The listing builds one solid part. Answer for the finished solid, in the listing's coordinates (mm). A direction names the side the tool comes from. Coordinates: 2 decimals unless noted, no trailing zeros. Loops run counter-clockwise (first coordinate to the right, second up) from the corner with the lowest first, then second, coordinate; pieces in that order, holes last. Notation, with made-up numbers: M 23,2 L 43,2 A22 cw 43,27 Z; hole C 88.5,27 d10. An arc over 180 degrees is marked long. Return JSON: item names as keys, results as strings. Group by question number.
1. Section A-A (z = 1.75) is taken. Write down the section's boundary in (x, y), then the cut area to 3 significant figures.
2. Which of the six approach directions +Z, -Z, +X, -X, +Y, -Y give full straight-line access (tool end or side, diameter ignored) to faces 1 (the face through (-83.949, 183.214, 5.239)), 2 (the face through (-84, 172.928, 6)), 3 (the face through (-82, 197.928, 6))?
3. Given P1, Ø5, axis at x = 86, z = 5.5, coming from the +Y side; P2, Ø2.5, axis at x = 46.78, y = 179.93, coming from the -Z side; P3, Ø5.5, axis at x = -53.42, y = 179.93, coming from the +Z side; P4, Ø0.9, axis at y = 171.5, z = 3.5, coming from the -X side, each flat-ended and moving along its own axis, determine where each tip first touches the part or whether it passes through.
4. Straight lines are drawn through the part: L1, parallel to Y at x = -83, z = 6; L2, parallel to Y at x = 19.5, z = 10.25; L3, parallel to X at y = 179, z = 6. For each, find the intervals that lie inside material, in ascending order. Write a range as from..to.
5. The mould has two halves that part along Y. Classify faces 4 (the face through (-78.019, 171, 6)), 5 (the face through (85, 197.928, 6)), 6 (the face through (87.311, 186.122, 5.785)): pulls with the +Y half, pulls with the -Y half, needs draft (parallel to the pull), parting line crosses it, or undercut.
```python
from build123d import *

# Parameters (mm, degrees)
ESBO_O1_W                                      = 119
ESBO_O1_H                                      = 30
RESSALTO_EXTRUS_O1_DEPTH                       = 12
ESCAREADO_PARA_SFHCS_M31_D                     = 3.4
ESCAREADO_PARA_SFHCS_M31_CSINK_D               = 6.72
ESCAREADO_PARA_SFHCS_M31_CSINK_ANGLE           = 90
ESBO_O8_W                                      = 26.2
ESBO_O8_H                                      = 30
RESSALTO_EXTRUS_O2_DEPTH                       = 12
ESBO_O9_W                                      = 36.2
ESBO_O9_H                                      = 30
RESSALTO_EXTRUS_O3_DEPTH                       = 12
ESBO_O10_W                                     = 12
ESBO_O10_H                                     = 12
CORTE_EXTRUS_O1_DEPTH                          = 2
FILETE1_R                                      = 2
ESBO_O12_W                                     = 11
ESBO_O12_H                                     = 12
CORTE_EXTRUS_O2_DEPTH                          = 3
BROCA_DE_ROSQUEAR_PARA_TARRAXA_DE_M4X0_7_D     = 3.3
BROCA_DE_ROSQUEAR_PARA_TARRAXA_DE_M4X0_7_DEPTH = 10
BROCA_DE_ROSQUEAR_PARA_TARRAXA_DE_M4X0_7_TIP   = 0.991420021
ESBO_O15_W                                     = 12
ESBO_O15_H                                     = 12
CORTE_EXTRUS_O3_DEPTH                          = 2
FILETE2_R                                      = 2
BROCA_DE_ROSQUEAR_PARA_TARRAXA_DE_M4_2_D       = 3.3
BROCA_DE_ROSQUEAR_PARA_TARRAXA_DE_M4_2_DEPTH   = 10
BROCA_DE_ROSQUEAR_PARA_TARRAXA_DE_M4_2_TIP     = 0.991420021


with BuildPart() as part:
    # Esboço1 → Ressalto-extrusão1 (new body)
    with BuildSketch(Plane.XY):
        with Locations((-3.319388577, 184.927849727)):
            Rectangle(ESBO_O1_W, ESBO_O1_H)
    extrude(amount=RESSALTO_EXTRUS_O1_DEPTH)

    # Escareado para SFHCS M31 (through all)
    with Locations(Plane.XY.offset(12)):
        with Locations((46.780611423, 179.927849727), (-53.419388577, 179.927849727), (-26.219388577, 179.927849727), (19.580611423, 179.927849727)):
            CounterSinkHole(ESCAREADO_PARA_SFHCS_M31_D / 2, ESCAREADO_PARA_SFHCS_M31_CSINK_D / 2, counter_sink_angle=ESCAREADO_PARA_SFHCS_M31_CSINK_ANGLE)

    # Esboço8 → Ressalto-extrusão2 (add)
    with BuildSketch(Plane.XY.offset(12)):
        with Locations((-75.919388577, 184.927849727)):
            Rectangle(ESBO_O8_W, ESBO_O8_H)
    extrude(amount=-RESSALTO_EXTRUS_O2_DEPTH)

    # Esboço9 → Ressalto-extrusão3 (add)
    with BuildSketch(Plane.XY):
        with Locations((74.280611423, 184.927849727)):
            Rectangle(ESBO_O9_W, ESBO_O9_H)
    extrude(amount=RESSALTO_EXTRUS_O3_DEPTH)

    # Esboço10 → Corte-extrusão1 (cut)
    with BuildSketch(Plane(origin=(0, 199.927849727, 0), x_dir=(1, 0, 0), z_dir=(0, 1, 0))):
        with Locations((-83.019388577, -6)):
            Rectangle(ESBO_O10_W, ESBO_O10_H)
    extrude(amount=-CORTE_EXTRUS_O1_DEPTH, mode=Mode.SUBTRACT)

    # Filete1
    filete1_edges = [part.edges().sort_by_distance(p)[0] for p in [
        (-89.019388577, 197.927849727, 6),
    ]]
    fillet(filete1_edges, radius=FILETE1_R)

    # Esboço12 → Corte-extrusão2 (cut)
    with BuildSketch(Plane.XZ.offset(-169.927849727)):
        with Locations((-83.519388577, 6)):
            Rectangle(ESBO_O12_W, ESBO_O12_H)
    extrude(amount=-CORTE_EXTRUS_O2_DEPTH, mode=Mode.SUBTRACT)

    # Broca de rosquear para tarraxa de M4x0.7
    with Locations(Plane.ZY.offset(89.019388577)):
        with Locations((6, 184.677849727)):
            Hole(BROCA_DE_ROSQUEAR_PARA_TARRAXA_DE_M4X0_7_D / 2, depth=BROCA_DE_ROSQUEAR_PARA_TARRAXA_DE_M4X0_7_DEPTH)
            with Locations((0, 0, -(BROCA_DE_ROSQUEAR_PARA_TARRAXA_DE_M4X0_7_DEPTH + BROCA_DE_ROSQUEAR_PARA_TARRAXA_DE_M4X0_7_TIP / 2))):  # 118° drill point
                Cone(0, BROCA_DE_ROSQUEAR_PARA_TARRAXA_DE_M4X0_7_D / 2, BROCA_DE_ROSQUEAR_PARA_TARRAXA_DE_M4X0_7_TIP, mode=Mode.SUBTRACT)

    # Esboço15 → Corte-extrusão3 (cut)
    with BuildSketch(Plane(origin=(0, 199.927849727, 0), x_dir=(-1, 0, 0), z_dir=(0, 1, 0))):
        with Locations((-86.380611423, 6)):
            Rectangle(ESBO_O15_W, ESBO_O15_H)
    extrude(amount=-CORTE_EXTRUS_O3_DEPTH, mode=Mode.SUBTRACT)

    # Filete2
    filete2_edges = [part.edges().sort_by_distance(p)[0] for p in [
        (92.380611423, 197.927849727, 6),
    ]]
    fillet(filete2_edges, radius=FILETE2_R)

    # Broca de rosquear para tarraxa de M4 2
    with Locations(Plane(origin=(92.380611423, 0, 0), x_dir=(0, 0, -1), z_dir=(1, 0, 0))):
        with Locations((-6, 184.4862903)):
            Hole(BROCA_DE_ROSQUEAR_PARA_TARRAXA_DE_M4_2_D / 2, depth=BROCA_DE_ROSQUEAR_PARA_TARRAXA_DE_M4_2_DEPTH)
            with Locations((0, 0, -(BROCA_DE_ROSQUEAR_PARA_TARRAXA_DE_M4_2_DEPTH + BROCA_DE_ROSQUEAR_PARA_TARRAXA_DE_M4_2_TIP / 2))):  # 118° drill point
                Cone(0, BROCA_DE_ROSQUEAR_PARA_TARRAXA_DE_M4_2_D / 2, BROCA_DE_ROSQUEAR_PARA_TARRAXA_DE_M4_2_TIP, mode=Mode.SUBTRACT)


solid = part.part
```
Worked out:
{
 "1": {"outline": "M -89.02,172.93 L -78.02,172.93 L -78.02,169.93 L 92.38,169.93 L 92.38,195.93 A2 ccw 90.38,197.93 L 80.38,197.93 L 80.38,199.93 L -77.02,199.93 L -77.02,197.93 L -87.02,197.93 A2 ccw -89.02,195.93 Z; hole C -53.42,179.93 d3.4; hole C -26.22,179.93 d3.4; hole C 19.58,179.93 d3.4; hole C 46.78,179.93 d3.4", "area": "5,320 mm^2"},
 "2": {"face 1": "-X", "face 2": "+Z, -Z, -X, -Y", "face 3": "+Z, -Z, -X, +Y"},
 "3": {"P1": "y = 197.93", "P2": "through", "P3": "z = 11.39", "P4": "x = -78.02"},
 "4": {"L1": "172.93..183.03, 186.33..197.93", "L2": "169.93..178.23, 181.63..199.93", "L3": "-89.02..-54.84, -51.99..-27.64, -24.79..18.16, 21.01..45.36, 48.21..92.38"},
 "5": {"face 4": "needs draft", "face 5": "pulls with the +Y half", "face 6": "undercut"}
}
